The model under review builds one solid part; all positions refer to its coordinate system, in mm. Face numbers are marked on the shaded views. A direction names the side the tool comes from. Coordinates: 2 decimals unless noted, no trailing zeros. Write each loop counter-clockwise with the first axis right and the second up, starting at its lowest first coordinate (ties: lowest second). Pieces come first, ordered by that corner, then holes.
1) For line 1 (Z direction, x = -317, y = 65); line 2 (X direction, y = 34, z = 63); line 3 (Y direction, x = -84, z = 18.5), list the stretches that pass through material, from the lowest coordinate up.
2) Mouldability with a two-part tool opening along Y and no side actions: class the marked faces 3, 4 and 5 as released by +Y, released by -Y, zero draft, split by the parting line, or undercut.
3) Add section D-D, the plane x = -82. State the section outline as (y, z) points, then the cut area to 3 significant figures.
4) Machinability: for the marked faces 1 and 2, which of the approach directions +Z, -Z, +X, -X, +Y, -Y give a long, thin tool a straight path to every point of the face, cutting with its end or side? Answer none if there is none.
5) For P1, Ø5, axis at x = -62, z = 55, coming from the +Y side; P2, Ø3, axis at x = -316.5, z = 65.5, coming from the -Y side; P3, Ø4, axis at y = -4, z = 92.5, coming from the -X side, all flat-tipped, find the tip position at first contact; note any pin that passes through.
6) Add section A-A, the plane x = -212. State the section outline as (y, z) points.
7) Add section C-C, the plane y = 50. State the section outline as (x, z) points.
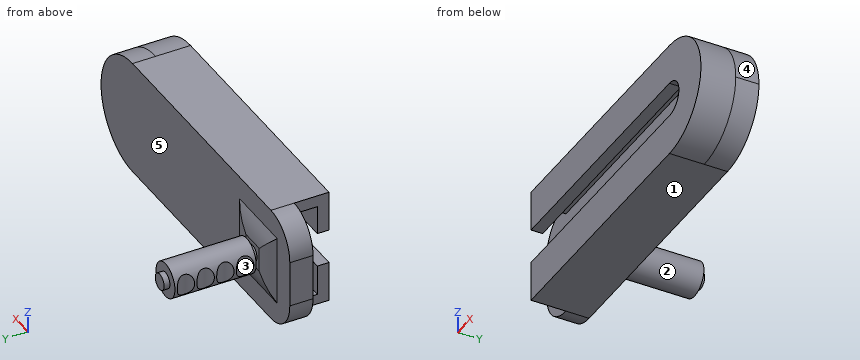
from build123d import *

# Parameters (mm, degrees)
SKETCH1_W           = 381
SKETCH1_H           = 127
BOSS_EXTRUDE1_DEPTH = 25.4
FILLET1_R           = 63.5
FILLET2_R           = 38.1
BOSS_EXTRUDE2_DEPTH = 25.4
BOSS_EXTRUDE3_DEPTH = 12.7
SKETCH4_W           = 76.2
SKETCH4_H           = 76.2
BOSS_EXTRUDE4_DEPTH = 6.35
FILLET3_R           = 50.8
SKETCH5_R           = 8.89
BOSS_EXTRUDE5_DEPTH = 6.35
SKETCH6_R           = 19.05
BOSS_EXTRUDE6_DEPTH = 88.9
CUT_EXTRUDE1_DEPTH  = 88.9
SKETCH8_R           = 8.89
BOSS_EXTRUDE7_DEPTH = 6.35
CUT_EXTRUDE2_START  = -12.7
CUT_EXTRUDE2_DEPTH  = 12.7
SKETCH10_R          = 5.08
CUT_EXTRUDE3_DEPTH  = 95.25


# Some blends are built 0.0001 mm under size
with BuildPart() as part:
    # Sketch1 → Boss-Extrude1 (new body)
    with BuildSketch(Plane(origin=(0, 0, 0), x_dir=(1, 0, 0), z_dir=(0, 1, 0))):
        with Locations((-190.5, -63.5)):
            Rectangle(SKETCH1_W, SKETCH1_H)
    extrude(amount=BOSS_EXTRUDE1_DEPTH)

    # Fillet1
    fillet1_edges = [part.edges().sort_by_distance(p)[0] for p in [
        (0, 12.7, 0),
        (0, 12.7, 127),
    ]]
    fillet(fillet1_edges, radius=FILLET1_R - 0.0001)  # a hair under: the kernel refuses the full size

    # Fillet2
    fillet2_edges = [part.edges().sort_by_distance(p)[0] for p in [
        (-381, 12.7, 127),
        (-381, 12.7, 0),
    ]]
    fillet(fillet2_edges, radius=FILLET2_R)

    # Sketch2 → Boss-Extrude2 (add)
    with BuildSketch(Plane(origin=(0, 0, 0), x_dir=(1, 0, 0), z_dir=(0, 1, 0))):
        with BuildLine():
            Line((-63.5, -12.7), (-342.9, -11.159231637))
            Line((-342.9, -11.159231637), (-342.9, 0))
            Line((-342.9, 0), (-63.5, 0))
            ThreePointArc((-63.5, 0), (0, -63.5), (-63.5, -127))
            Line((-63.5, -127), (-342.9, -127))
            Line((-342.9, -127), (-342.9, -114.3))
            Line((-342.9, -114.3), (-63.5, -114.3))
            ThreePointArc((-63.5, -114.3), (-12.7, -63.5), (-63.5, -12.7))
        make_face()
    extrude(amount=-BOSS_EXTRUDE2_DEPTH)

    # Sketch3 → Boss-Extrude3 (add)
    with BuildSketch(Plane(origin=(0, -25.4, 0), x_dir=(1, 0, 0), z_dir=(0, 1, 0))):
        with BuildLine():
            Line((-342.9, -127), (-342.9, -82.55))
            Line((-342.9, -82.55), (-63.5, -82.55))
            ThreePointArc((-63.5, -82.55), (-44.45, -63.5), (-63.5, -44.45))
            Line((-63.5, -44.45), (-342.9, -44.45))
            Line((-342.9, -44.45), (-342.9, 0))
            Line((-342.9, 0), (-63.5, 0))
            ThreePointArc((-63.5, 0), (0, -63.5), (-63.5, -127))
            Line((-63.5, -127), (-342.9, -127))
        make_face()
    extrude(amount=-BOSS_EXTRUDE3_DEPTH)

    # Sketch4 → Boss-Extrude4 (add)
    with BuildSketch(Plane(origin=(0, 25.4, 0), x_dir=(1, 0, 0), z_dir=(0, 1, 0))):
        with Locations((-317.5, -63.5)):
            Rectangle(SKETCH4_W, SKETCH4_H)
    extrude(amount=BOSS_EXTRUDE4_DEPTH)

    # Fillet3
    # the kernel refuses this fillet: 50.8 mm, written as the material it takes off along each edge
    with BuildSketch(Plane(origin=(-279.4, 31.75, 163.083610621), x_dir=(0, -1, 0), z_dir=(0, 0, -1)), Plane(origin=(-417.083610621, 31.75, 101.6), x_dir=(0, -1, 0), z_dir=(1, 0, 0)), Plane(origin=(-355.6, 31.75, -36.083610621), x_dir=(0, -1, 0), z_dir=(0, 0, 1)), Plane(origin=(-217.916389379, 31.75, 25.4), x_dir=(0, -1, 0), z_dir=(-1, 0, 0))) as fillet3_piece_1:
        with BuildLine():
            CenterArc((50.8, 24.593444248), FILLET3_R, 180, 28.955024372)
            Line((0, 24.593444248), (-1.016, 24.593444248))
            Line((-1.016, 24.593444248), (-1.016, 0))
            Line((-1.016, 0), (0, -1.016))
            ThreePointArc((0, -1.016), (3.175, -1.016), (5.461, -0.491868885))
            Line((5.461, -0.491868885), (6.35, 0))
        make_face()
    extrude(amount=199.167221242, mode=Mode.SUBTRACT)

    # Sketch5 → Boss-Extrude5 (add)
    with BuildSketch(Plane(origin=(0, 31.75, 0), x_dir=(1, 0, 0), z_dir=(0, 1, 0))):
        with Locations(Location((-317.5, -63.5, 0), (0, 0, 90))):
            Circle(SKETCH5_R)
    extrude(amount=BOSS_EXTRUDE5_DEPTH)

    # Sketch6 → Boss-Extrude6 (add)
    with BuildSketch(Plane(origin=(0, 38.1, 0), x_dir=(1, 0, 0), z_dir=(0, 1, 0))):
        with Locations(Location((-317.5, -63.5, 0), (0, 0, 270))):
            Circle(SKETCH6_R)
    extrude(amount=BOSS_EXTRUDE6_DEPTH)

    # Sketch7 → Cut-Extrude1 (cut)
    with BuildSketch(Plane.XY):
        with BuildLine():
            Line((-336.55, 127), (-336.55, 124.46))
            ThreePointArc((-336.55, 124.46), (-332.607071488, 114.940928512), (-336.55, 105.421857023))
            Line((-336.55, 105.421857023), (-336.55, 105.41))
            Line((-336.55, 105.41), (-336.55, 102.87))
            ThreePointArc((-336.55, 102.87), (-332.607071488, 93.350928512), (-336.55, 83.831857023))
            Line((-336.55, 83.831857023), (-336.55, 83.82))
            Line((-336.55, 83.82), (-336.55, 81.28))
            ThreePointArc((-336.55, 81.28), (-332.607071488, 71.760928512), (-336.55, 62.241857023))
            Line((-336.55, 62.241857023), (-336.55, 62.23))
            Line((-336.55, 62.23), (-336.55, 59.69))
            ThreePointArc((-336.55, 59.69), (-332.607071488, 50.170928512), (-336.55, 40.651857023))
            Line((-336.55, 40.651857023), (-336.55, 40.64))
            Line((-336.55, 40.64), (-368.013875858, 40.64))
            Line((-368.013875858, 40.64), (-368.013875858, 127.710007378))
            Line((-368.013875858, 127.710007378), (-336.55, 127))
        make_face()
    extrude(amount=CUT_EXTRUDE1_DEPTH, mode=Mode.SUBTRACT)

    # Sketch8 → Boss-Extrude7 (add)
    with BuildSketch(Plane(origin=(0, 127, 0), x_dir=(1, 0, 0), z_dir=(0, 1, 0))):
        with Locations(Location((-317.5, -63.5, 0), (0, 0, 90))):
            Circle(SKETCH8_R)
    extrude(amount=BOSS_EXTRUDE7_DEPTH)

    # Sketch9 → Cut-Extrude2 (cut)
    with BuildSketch(Plane.XZ.offset(CUT_EXTRUDE2_START)):
        with BuildLine():
            Line((-342.9, 82.55), (-63.5, 82.55))
            ThreePointArc((-63.5, 82.55), (-44.45, 63.5), (-63.5, 44.45))
            Line((-63.5, 44.45), (-342.9, 44.45))
            Line((-342.9, 44.45), (-342.9, 82.55))
        make_face()
    extrude(amount=CUT_EXTRUDE2_DEPTH, mode=Mode.SUBTRACT)

    # Sketch10 → Cut-Extrude3 (cut)
    with BuildSketch(Plane.XZ.offset(-12.7)):
        with Locations(Location((-317.5, 63.5, 0), (0, 0, 270))):
            Circle(SKETCH10_R)
    extrude(amount=-CUT_EXTRUDE3_DEPTH, mode=Mode.SUBTRACT)


solid = part.part
Geometry results:
1. line 1: z = 44.46 to 58.44, 68.56 to 82.54
1. line 2: x = -326.38 to -322.56, -312.44 to -308.62
1. line 3: y = -38.1 to -25.4, 0 to 25.4
2. face 3: undercut
2. face 4: zero draft
2. face 5: released by +Y
3. outline: (-38.1, 0) - (25.4, 0) - (25.4, 127) - (-38.1, 127) - (-38.1, 82.55) - (-25.4, 82.55) - (-25.4, 114.3) - (0, 114.3) - (0, 82.55) - (12.7, 82.55) - (12.7, 44.45) - (0, 44.45) - (0, 12.6) - (-25.4, 12.6) - (-25.4, 44.45) - (-38.1, 44.45) - close
3. area: 4,510 mm2
4. face 1: -Z, +X, -X, +Y, -Y
4. face 2: +Y
5. P1: stops at y = 25.4
5. P2: stops at y = 107.95
5. P3: stops at x = -23.26
6. outline: (-38.1, 0) - (25.4, 0) - (25.4, 127) - (-38.1, 127) - (-38.1, 82.55) - (-25.4, 82.55) - (-25.4, 114.3) - (0, 114.3) - (0, 82.55) - (12.7, 82.55) - (12.7, 44.45) - (0, 44.45) - (0, 11.88) - (-25.4, 11.88) - (-25.4, 44.45) - (-38.1, 44.45) - close
7. outline: (-332.61, 51.9) arc R19.05 ccw (long way) to (-332.61, 75.1) - close; hole circle Ø10.16 at (-317.5, 63.5)
